```python
from build123d import *

# Parameters (mm, degrees)
SKETCH1_R                       = 2.9
BOSS_EXTRUDE1_DEPTH             = 15
SKETCH2_R                       = 1
CUT_EXTRUDE1_DEPTH              = 16
TAP_DRILL_FOR_M3X0_5_TAP1_D     = 2.5
TAP_DRILL_FOR_M3X0_5_TAP1_DEPTH = 11
TAP_DRILL_FOR_M3X0_5_TAP1_TIP   = 0.751075774
SKETCH5_W                       = 3
SKETCH5_H                       = 1.793791595
CHAMFER1_SIZE                   = 0.75
CHAMFER1_SIZE2                  = 1.299038106
CHAMFER2_SIZE                   = 1.21
CHAMFER2_SIZE2                  = 0.698593826


with BuildPart() as part:
    # Sketch1 → Boss-Extrude1 (new body)
    with BuildSketch(Plane.XY):
        Circle(SKETCH1_R)
    extrude(amount=BOSS_EXTRUDE1_DEPTH)

    # Sketch2 → Cut-Extrude1 (cut, through all)
    with BuildSketch(Plane(origin=(0, 0, 0), x_dir=(-1, 0, 0), z_dir=(0, 0, -1))):
        Circle(SKETCH2_R)
    extrude(amount=-CUT_EXTRUDE1_DEPTH, mode=Mode.SUBTRACT)

    # Tap Drill for M3x0.5 Tap1
    with Locations(Plane(origin=(0, 0, 0), x_dir=(-1, 0, 0), z_dir=(0, 0, -1))):
        with Locations((0, 0)):
            Hole(TAP_DRILL_FOR_M3X0_5_TAP1_D / 2, depth=TAP_DRILL_FOR_M3X0_5_TAP1_DEPTH)
            with Locations((0, 0, -(TAP_DRILL_FOR_M3X0_5_TAP1_DEPTH + TAP_DRILL_FOR_M3X0_5_TAP1_TIP / 2))):  # 118° drill point
                Cone(0, TAP_DRILL_FOR_M3X0_5_TAP1_D / 2, TAP_DRILL_FOR_M3X0_5_TAP1_TIP, mode=Mode.SUBTRACT)

    # Sketch5 → Cut-Revolve1 (revolve, cut)
    with BuildSketch(Plane(origin=(0, 0, 0), x_dir=(0, 0, -1), z_dir=(1, 0, 0))):
        with Locations((-12.5, 2.896895798)):
            Rectangle(SKETCH5_W, SKETCH5_H)
    revolve(axis=Axis((0, 0, 0), (0, 0, 1)), mode=Mode.SUBTRACT)

    # Chamfer1
    chamfer1_edges = [part.edges().sort_by_distance(p)[0] for p in [
        (-1.25, 0, 0),
    ]]
    chamfer1_side = [part.faces().sort_by_distance(p)[0] for p in [
        (-2.817975613, 0, 0),
    ]]
    chamfer(chamfer1_edges, length=CHAMFER1_SIZE, length2=CHAMFER1_SIZE2, reference=chamfer1_side[0])

    # Chamfer2
    chamfer2_edges = [part.edges().sort_by_distance(p)[0] for p in [
        (1, 0, 15),
    ]]
    chamfer2_side = [part.faces().sort_by_distance(p)[0] for p in [
        (1, 0, 13.075107577),
    ]]
    chamfer(chamfer2_edges, length=CHAMFER2_SIZE, length2=CHAMFER2_SIZE2, reference=chamfer2_side[0])


solid = part.part
```
Can you work these out from the model? Positions are in its coordinate system, mm. A direction names the side the tool comes from. Round coordinates to 2 decimals unless told otherwise and drop trailing zeros. Loops run counter-clockwise (first coordinate to the right, second up) from the corner with the lowest first, then second, coordinate; pieces in that order, holes last. Notation, with made-up numbers: M 82.25,45.25 L 86.25,45.25 A25 ccw 86.25,71.25 Z; hole C 30,45.25 d7. An arc over 180 degrees is marked long. Write item = value, one per line. Start each with the question number.
(1) Suppose I cut it at A-A on y = 0. Write out the boundary of the cut face in (x, z), plus the area to 3 significant figures.
(2) I'm going to push flat-ended pins straight in: P1, Ø1, axis at y = -1, z = 13, coming from the +X side; P2, Ø3, axis at x = 0, y = 0, coming from the +Z side; P3, Ø3, axis at x = 0, y = 0, coming from the -Z side. Where does each tip first touch, or does it pass through?
(3) If we mould it in two halves opening along Z, with no side actions, what happens to faces 1 (the face through (0, -2, 15)), 2 (the face through (-1, -2, 0)), 3 (the face through (-1, -2, 14)), 4 (the face through (-0.27, -1.22, 6.22))? For each: released by +Z, released by -Z, zero draft, split by the parting line, or undercut.
(4) Which directions (+Z, -Z, +X, -X, +Y, -Y) give clear straight access to the entire face, cutting with the end or side of a thin tool? Please do faces 5 (the face through (-2.9, 0.1, 5.4)), 6 (the face through (-2, 0, 12)).
(5) I need wall thicknesses on line 1 along Z through (x, y) = (-2, 1); line 2 along X through (y, z) = (0, 12.5); line 3 along Y through (x, z) = (0, 8). Which ranges of each line are inside material? Lowest first, please.
(6) Suppose I cut it at C-C on z = 9.5. Write out the boundary of the cut face in (x, y).
Answer block:
q1.outline = M -2.9,0 L -2,0 L -1.25,1.3 L -1.25,11 L -1,11.15 L -1,13.79 L -1.7,15 L -2.9,15 L -2.9,14 L -2,14 L -2,11 L -2.9,11 Z; M 1,11.15 L 1.25,11 L 1.25,1.3 L 2,0 L 2.9,0 L 2.9,11 L 2,11 L 2,14 L 2.9,14 L 2.9,15 L 1.7,15 L 1,13.79 Z
q1.area = 44.2 mm²
q2.P1 = 1.94
q2.P2 = 14.66
q2.P3 = 0.87
q3.face_1 = released by +Z
q3.face_2 = released by -Z
q3.face_3 = undercut
q3.face_4 = zero draft
q4.face_5 = +Z, -Z
q4.face_6 = none
q5.line_1 = 0 to 11, 14 to 15
q5.line_2 = -2 to -1, 1 to 2
q5.line_3 = -2.9 to -1.25, 1.25 to 2.9
q6.outline = C 0,0 d5.8; hole C 0,0 d2.5
